from build123d import *

# Parameters (mm, degrees)
SKETCH1_W           = 112.6
SKETCH1_H           = 40.72
BOSS_EXTRUDE1_DEPTH = 6.35
SKETCH2_W           = 112.6
SKETCH2_H           = 6.35
BOSS_EXTRUDE2_DEPTH = 56
SKETCH3_W           = 60
SKETCH3_H           = 56
SKETCH3_W_2         = 54.5
SKETCH3_H_2         = 50.5
BOSS_EXTRUDE3_DEPTH = 15


with BuildPart() as part:
    # Sketch1 → Boss-Extrude1 (new body)
    with BuildSketch(Plane(origin=(0, 0, 0), x_dir=(1, 0, 0), z_dir=(0, 1, 0))):
        Rectangle(SKETCH1_W, SKETCH1_H)
    extrude(amount=BOSS_EXTRUDE1_DEPTH)

    # Sketch2 → Boss-Extrude2 (add)
    with BuildSketch(Plane.XY.offset(20.36)):
        with Locations((0, 3.175)):
            Rectangle(SKETCH2_W, SKETCH2_H)
    extrude(amount=BOSS_EXTRUDE2_DEPTH)

    # Sketch3 → Boss-Extrude3 (add)
    with BuildSketch(Plane(origin=(0, 6.35, 0), x_dir=(1, 0, 0), z_dir=(0, 1, 0))):
        with Locations((26.3, -48.36)):
            Rectangle(SKETCH3_W, SKETCH3_H)
        with Locations((26.3, -48.36)):
            Rectangle(SKETCH3_W_2, SKETCH3_H_2, mode=Mode.SUBTRACT)
    extrude(amount=BOSS_EXTRUDE3_DEPTH)


solid = part.part
The model under review builds one solid part; all positions refer to its coordinate system, in mm. A direction names the side the tool comes from. Round coordinates to 2 decimals unless told otherwise and drop trailing zeros. Write each loop counter-clockwise with the first axis right and the second up, starting at its lowest first coordinate (ties: lowest second). Pieces come first, ordered by that corner, then holes. Notation, with made-up numbers: (-26.75, 80) - (29.25, 80) arc R31 ccw to (29.25, 104) - close; hole circle Ø8 at (-11, 58.25). An arc over 180 degrees is marked (long way). One line per item, written item: value. Start each with the question number.
1. To check wall thickness, follow L1, parallel to X at y = 15, z = 59; L2, parallel to Z at x = 14, y = 17.25; L3, parallel to Y at x = 2, z = 15. State the ranges of each line that lie inside material, in increasing order. Write a range as from..to.
2. Clearance check with flat-ended pins moving along their axes: P1, Ø12, axis at y = 16.5, z = 53, coming from the -X side; P2, Ø1.5, axis at x = -28, z = 62, coming from the +Y side; P3, Ø4.5, axis at x = 25, y = 11, coming from the -Z side. State where each tip first meets the part, or that it passes through.
3. Consider section A-A on z = 25.5. Write out the cut boundary in (x, y), and give its area (3 significant figures).
4. Machinability: for faces 1 (the face through (26, 14, 20.36)), 2 (the face through (-3.7, 14, 49)), 3 (the face through (26, 6.35, 48)), which of the approach directions +Z, -Z, +X, -X, +Y, -Y give a long, thin tool a straight path to every point of the face, cutting with its end or side? Answer none if there is none.
5. Consider section B-B on y = 19.75. Write out the cut boundary in (x, z), and give its area (3 significant figures).
6. The part is to be moulded in two halves that separate along X. For faces 4 (the face through (53.55, 14, 49)), 5 (the face through (12, 8, 76.36)), 6 (the face through (56.3, 8, 39)), 7 (the face through (-56.3, 3, 27)), say which applies: released by +X, released by -X, zero draft, split by the parting line, or undercut.
7. Consider section C-C on x = 48.5. Write out the cut boundary in (y, z), and give its area (3 significant figures).
8. Consider section D-D on z = 8.5. Write out the cut boundary in (x, y), and give its area (3 significant figures).
Checks:
1. L1: x = -3.7..-0.95, 53.55..56.3
1. L2: z = 20.36..23.11, 73.61..76.36
1. L3: y = 0..6.35
2. P1: stops at x = -3.7
2. P2: stops at y = 6.35
2. P3: stops at z = 20.36
3. outline: (-56.3, 0) - (56.3, 0) - (56.3, 21.35) - (53.55, 21.35) - (53.55, 6.35) - (-0.95, 6.35) - (-0.95, 21.35) - (-3.7, 21.35) - (-3.7, 6.35) - (-56.3, 6.35) - close
3. area: 798 mm^2
4. face 1: -Z, +X, -X, +Y
4. face 2: +Z, -Z, -X, +Y
4. face 3: +Y
5. outline: (-3.7, 20.36) - (56.3, 20.36) - (56.3, 76.36) - (-3.7, 76.36) - close; hole (-0.95, 23.11) - (53.55, 23.11) - (53.55, 73.61) - (-0.95, 73.61) - close
5. area: 608 mm^2
6. face 4: undercut
6. face 5: zero draft
6. face 6: released by +X
6. face 7: released by -X
7. outline: (0, -20.36) - (6.35, -20.36) - (6.35, 20.36) - (21.35, 20.36) - (21.35, 23.11) - (6.35, 23.11) - (6.35, 73.61) - (21.35, 73.61) - (21.35, 76.36) - (0, 76.36) - close
7. area: 697 mm^2
8. outline: (-56.3, 0) - (56.3, 0) - (56.3, 6.35) - (-56.3, 6.35) - close
8. area: 715 mm^2
